Check sheet for the modelled part. Datum: model origin and axes. Units: mm. A direction names the side the tool comes from. Coordinates: 2 decimals unless noted, no trailing zeros. Loops run counter-clockwise (first coordinate to the right, second up) from the corner with the lowest first, then second, coordinate; pieces in that order, holes last. Notation, with made-up numbers: (22, 79) - (69, 79) arc R25 cw to (69, 102) - close; hole circle Ø5 at (60, -24.75). An arc over 180 degrees is marked (long way). Use a Markdown table: item, result. Add a question column.
1) Go/stop test with flat-tipped pins: P1, Ø4, axis at y = 101.5, z = 7, coming from the -X side; P2, Ø3, axis at y = 156.5, z = 9, coming from the -X side; P3, Ø1.5, axis at y = 147, z = -6.5, coming from the +X side. Record where each tip stops, or that it passes through.
2) Tool access check on faces 4 (the cylindrical face through (-13.566, 90.145, 7.056)), 5 (the conical face through (-18.704, 147.575, -4.153)). Record the directions out of +Z, -Z, +X, -X, +Y, -Y that give a thin tool (end or side, any length) a straight path to the whole face; none if there is none.
3) Sectioned sample at A-A, the plane y = 68.5. Enter the section's corners in (x, z), then the cut area to 3 significant figures.
4) Draft check along Y on faces 1 (the flat face through (-15.5, 0, 1.5)), 2 (the flat face through (-15.5, 177.8, -1.5)), 3 (the conical face through (-18.704, 37.975, -4.153)). Enter one of: pulls with the +Y half, pulls with the -Y half, needs draft (parallel to the pull), parting line crosses it, or undercut.
5) Thickness scan on line 1 (X direction, y = 66, z = 0); line 2 (Z direction, x = -9, y = 144.5); line 3 (Z direction, x = 2, y = 64). Record the ranges inside material, lowest first.
from build123d import *


with BuildPart() as part:
    # Sketch1 → Revolve1 (revolve)
    with BuildSketch(Plane(origin=(0, 0, 0), x_dir=(-1, 0, 0), z_dir=(0, 0, -1)), mode=Mode.PRIVATE) as revolve1_sk:
        Polygon((-15.2908, 177.8), (-21.034375, 177.8), (-21.034375, 149.7), (-19.034375, 147.7), (-21.034375, 145.7), (-21.034375, 141.7), (-19.034375, 139.7), (-21.034375, 137.7), (-21.034375, 133.7), (-19.034375, 131.7), (-21.034375, 129.7), (-21.034375, 88.9), (-21.034375, 48.1), (-19.034375, 46.1), (-21.034375, 44.1), (-21.034375, 40.1), (-19.034375, 38.1), (-21.034375, 36.1), (-21.034375, 32.1), (-19.034375, 30.1), (-21.034375, 28.1), (-21.034375, 0), (-15.2908, 0), align=None)
    revolve(revolve1_sk.sketch.rotate(Axis((0, 0, 0), (0, 1, 0)), 270), axis=Axis((0, 0, 0), (0, 1, 0)))


solid = part.part
Solved:
| question | item | result |
|---|---|---|
| 1 | P1 | stops at x = -20.43 |
| 1 | P2 | stops at x = -19.65 |
| 1 | P3 | stops at x = 19.46 |
| 2 | face 4 | +Y, -Y |
| 2 | face 5 | none |
| 3 | outline | circle Ø42.07 at (0, 0); hole circle Ø30.58 at (0, 0) |
| 3 | area | 655 mm2 |
| 4 | face 1 | pulls with the -Y half |
| 4 | face 2 | pulls with the +Y half |
| 4 | face 3 | undercut |
| 5 | line 1 | x = -21.03 to -15.29, 15.29 to 21.03 |
| 5 | line 2 | z = -19.01 to -12.36, 12.36 to 19.01 |
| 5 | line 3 | z = -20.94 to -15.16, 15.16 to 20.94 |
